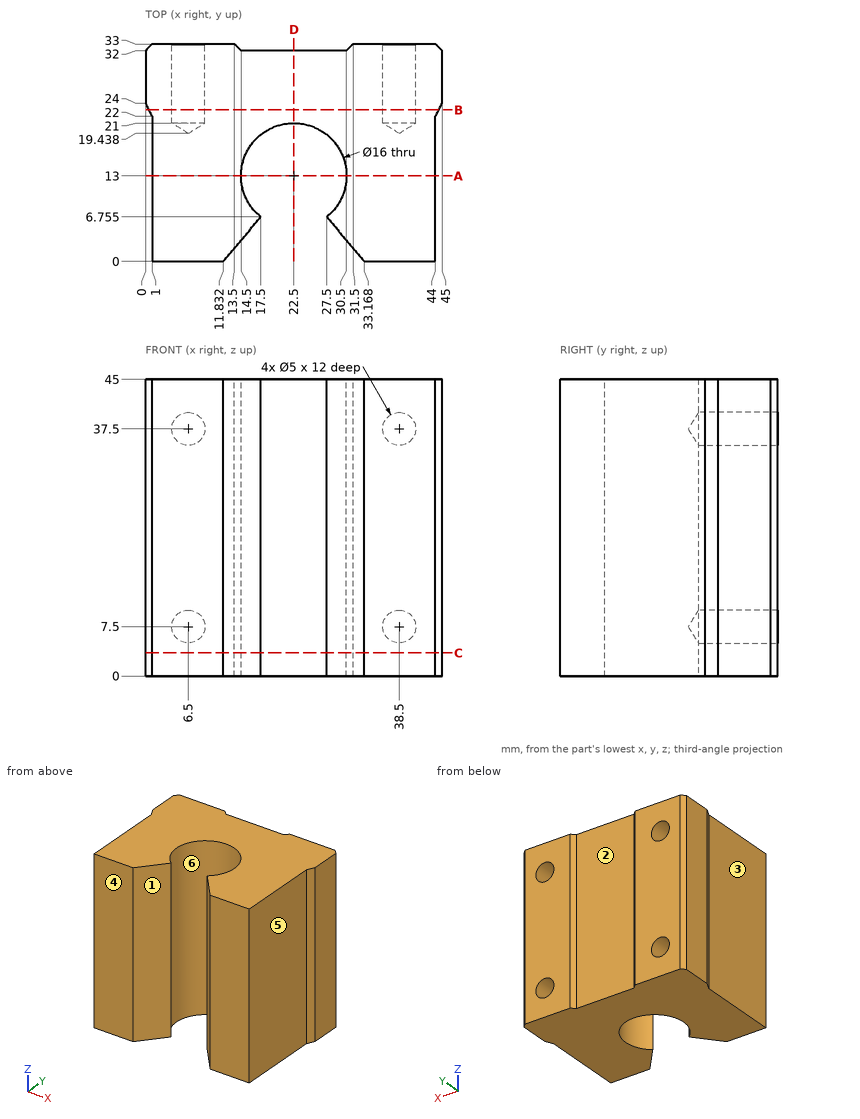
Geometry check sheet. Reference: drawing and pictorial views, mm from the part's lowest x, y, z. A direction names the side the tool comes from. Give positions to 0.01 mm unless a question says otherwise; leave off trailing zeros. Loops run counter-clockwise (first coordinate to the right, second up) from the corner with the lowest first, then second, coordinate; pieces in that order, holes last.
1. Section check C-C, the plane z = 3.5. Enter the section's corners in (x, y) (3 decimals), then the cut area to 3 significant figures.
2. Mould release check, pull along Y, two halves, no side actions. Record for the marked faces 4, 5 and 6: released by +Y, released by -Y, zero draft, split by the parting line, or undercut.
3. Go/stop test with flat-tipped pins: pin 1 Ø6 at (x, z) = (38.5, 37.5) entering from +Y; pin 2 Ø4.5 at (x, z) = (6.5, 37.5) entering from +Y; pin 3 Ø4 at (x, z) = (6.5, 7.5) entering from +Y; pin 4 Ø3 at (y, z) = (9, 22.5) entering from -X. Record where each tip stops, or that it passes through.
4. Section check A-A, the plane y = 13. Enter the section's corners in (x, z).
5. Set-up check for the marked faces 1, 2 and 3: record each of +Z, -Z, +X, -X, +Y, -Y from which the full face is reachable in a straight line by a thin tool's end or side.
6. Section check B-B, the plane y = 23. Enter the section's corners in (x, z), then the cut area to 3 significant figures.
7. Section check D-D, the plane x = 22.5. Enter the section's corners in (y, z), then the cut area to 3 significant figures.
8. Thickness scan on line 1 (X direction, y = 26, z = 7.5); line 2 (Z direction, x = 38, y = 28); line 3 (X direction, y = 23.5, z = 37.5). Record the ranges inside material, lowest first.
Geometry says:
1. outline: (0, 24) - (1, 22) - (1, 0) - (11.832, 0) - (17.5, 6.755) arc R8 cw (long way) to (27.5, 6.755) - (33.168, 0) - (44, 0) - (44, 22) - (45, 24) - (45, 32) - (44, 33) - (31.5, 33) - (30.5, 32) - (14.5, 32) - (13.5, 33) - (1, 33) - (0, 32) - close
1. area: 1,130 mm2
2. face 4: released by -Y
2. face 5: zero draft
2. face 6: undercut
3. pin 1: stops at y = 33
3. pin 2: stops at y = 20.84
3. pin 3: stops at y = 20.69
3. pin 4: stops at x = 1
4. outline: (1, 0) - (14.5, 0) - (14.5, 45) - (1, 45) - close; (30.5, 0) - (44, 0) - (44, 45) - (30.5, 45) - close
5. face 1: +Z, -Z, -Y
5. face 2: +Z, -Z, +Y
5. face 3: +Z, -Z, -X, -Y
6. outline: (0.5, 0) - (44.5, 0) - (44.5, 45) - (0.5, 45) - close; hole circle Ø5 at (6.5, 7.5); hole circle Ø5 at (6.5, 37.5); hole circle Ø5 at (38.5, 7.5); hole circle Ø5 at (38.5, 37.5)
6. area: 1,900 mm2
7. outline: (21, 0) - (32, 0) - (32, 45) - (21, 45) - close
7. area: 495 mm2
8. line 1: x = 0 to 4, 9 to 36, 41 to 45
8. line 2: z = 0 to 5.05, 9.95 to 35.05, 39.95 to 45
8. line 3: x = 0.25 to 4, 9 to 36, 41 to 44.75
